```python
from build123d import *

# Parameters (mm, degrees)
SKETCH2_W                                   = 101.6
SKETCH2_H                                   = 127
BOSS_EXTRUDE1_DEPTH                         = 3.175
SKETCH5_R                                   = 3.9751
CUT_EXTRUDE1_DEPTH                          = 3.175
BOSS_EXTRUDE3_DEPTH                         = 92.87256
BOSS_EXTRUDE4_DEPTH                         = 6.35
SKETCH18_R                                  = 3.175
CUT_EXTRUDE3_DEPTH                          = 6.8072
FILLET4_R                                   = 4.0005
CUT_EXTRUDE4_DEPTH                          = 34.5948
CUT_EXTRUDE5_DEPTH                          = 2.9972
FILLET7_R                                   = 2.54
CSK_FOR_1_4_FLAT_HEAD_MACHINE_SCREW_2_COUNT = 2
CSK_FOR_1_4_FLAT_HEAD_MACHINE_SCREW_2_PITCH = 55.9


with BuildPart() as part:
    # Sketch2 → Boss-Extrude1 (new body)
    with BuildSketch(Plane.XY):
        with Locations((50.8, 63.5)):
            Rectangle(SKETCH2_W, SKETCH2_H)
    extrude(amount=BOSS_EXTRUDE1_DEPTH)

    # Sketch5 → Cut-Extrude1 (cut)
    with BuildSketch(Plane(origin=(0, 0, 0), x_dir=(-1, 0, 0), z_dir=(0, 0, -1))):
        with BuildLine():
            Line((-81.586228812, 65.152573183), (-58.571239337, 65.152573183))
            ThreePointArc((-58.571239337, 65.152573183), (-49.65943867, 58.729036089), (-53.287760408, 48.359981104))
            ThreePointArc((-53.287760408, 48.359981104), (-57.249364207, 28.049269577), (-36.93865268, 24.087665778))
            ThreePointArc((-36.93865268, 24.087665778), (-28.337713232, 24.971703827), (-22.817162059, 18.317291951))
            ThreePointArc((-22.817162059, 18.317291951), (-16.509170131, 7.896881921), (-5.03428, 3.81))
            Line((-5.03428, 3.81), (-5.03428, 0))
            Line((-5.03428, 0), (0, 0))
            Line((0, 0), (0, 127))
            Line((0, 127), (-101.6, 127))
            Line((-101.6, 127), (-101.6, 0))
            Line((-101.6, 0), (-97.90684, 0))
            Line((-97.90684, 0), (-97.90684, 65.152573183))
            Line((-97.90684, 65.152573183), (-81.586228812, 65.152573183))
        make_face()
        with Locations((-58.416247506, 55.973867932)):
            Circle(SKETCH5_R)
        with Locations((-31.810165582, 16.473778949)):
            Circle(SKETCH5_R)
    extrude(amount=-CUT_EXTRUDE1_DEPTH, mode=Mode.SUBTRACT)

    # Sketch10 → Boss-Extrude3 (add)
    with BuildSketch(Plane(origin=(5.03428, 0, 0), x_dir=(0, 0, -1), z_dir=(1, 0, 0))):
        Polygon((-3.175, 0), (-4.2418, 0), (-4.2418, -2.9972), (-34.5948, -2.9972), (-34.5948, 0), (-34.5948, 3.81), (-3.175, 3.81), align=None)
    extrude(amount=BOSS_EXTRUDE3_DEPTH)

    # Sketch11 → Boss-Extrude4 (add)
    with BuildSketch(Plane(origin=(97.90684, 0, 0), x_dir=(0, 0, -1), z_dir=(1, 0, 0))):
        Polygon((-3.175, 65.152573183), (-3.175, 3.81), (-34.5948, 3.81), align=None)
    extrude(amount=-BOSS_EXTRUDE4_DEPTH)

    # Sketch18 → Cut-Extrude3 (cut)
    with BuildSketch(Plane.XZ.offset(2.9972)):
        with Locations(Location((25.968032816, 23.228300068, 0), (0, 0, 270))):
            Circle(SKETCH18_R)
        with Locations(Location((81.868032816, 23.228300068, 0), (0, 0, 270))):
            Circle(SKETCH18_R)
    extrude(amount=-CUT_EXTRUDE3_DEPTH, mode=Mode.SUBTRACT)

    # Fillet4
    fillet4_edges = [part.edges().sort_by_distance(p)[0] for p in [
        (97.90684, -1.4986, 4.2418),
        (5.03428, -1.4986, 4.2418),
        (97.90684, 0.4064, 34.5948),
        (5.03428, 0.4064, 34.5948),
    ]]
    fillet(fillet4_edges, radius=FILLET4_R)

    # Mirror5: part across plane


with BuildPart() as part_1:
    add(part.part)
    add(part.part.mirror(Plane.XY))

    # Sketch25 → Cut-Extrude4 (cut)
    with BuildSketch(Plane.XY):
        Polygon((105.475480197, -15.241589329), (106.840773124, 71.833759528), (-8.541984089, 73.642896836), (-9.907277015, -13.432452021), align=None)
    extrude(amount=CUT_EXTRUDE4_DEPTH, mode=Mode.SUBTRACT)

    # Sketch28 → Cut-Extrude5 (cut)
    with BuildSketch(Plane.XZ.offset(2.9972)):
        with BuildLine():
            Line((93.90634, -4.2418), (9.03478, -4.2418))
            ThreePointArc((9.03478, -4.2418), (6.205999322, -5.413519322), (5.03428, -8.2423))
            Line((5.03428, -8.2423), (5.03428, -30.5943))
            ThreePointArc((5.03428, -30.5943), (6.205999322, -33.423080678), (9.03478, -34.5948))
            Line((9.03478, -34.5948), (93.90634, -34.5948))
            ThreePointArc((93.90634, -34.5948), (96.735120678, -33.423080678), (97.90684, -30.5943))
            Line((97.90684, -30.5943), (97.90684, -8.2423))
            ThreePointArc((97.90684, -8.2423), (96.735120678, -5.413519322), (93.90634, -4.2418))
        make_face()
    extrude(amount=-CUT_EXTRUDE5_DEPTH, mode=Mode.SUBTRACT)

    # Fillet7
    # the kernel refuses this fillet: 2.54 mm, written as the material it adds along each edge
    with BuildSketch(Plane(origin=(89.01684, 6.35, -5.715), x_dir=(0, -1, 0), z_dir=(1, 0, 0))) as fillet7_piece_1_section:
        Polygon((0, 0), (FILLET7_R, 0), (FILLET7_R, -FILLET7_R), (0, -FILLET7_R), align=None)
    fillet7_piece_1 = extrude(amount=FILLET7_R, mode=Mode.PRIVATE)
    fillet7_piece_1 = fillet7_piece_1 - Plane(origin=(89.01684, 6.35, -5.715), x_dir=(0, 0.7071067811865475, -0.7071067811865477), z_dir=(1, 0, 0)) * Sphere(FILLET7_R, mode=Mode.PRIVATE)
    add(fillet7_piece_1)
    with BuildSketch(Plane(origin=(5.03428, 3.81, -3.175), x_dir=(0, 0, -1), z_dir=(1, 0, 0))) as fillet7_piece_2_section:
        with BuildLine():
            CenterArc((FILLET7_R, FILLET7_R), FILLET7_R, 180, 90)
            Line((0, FILLET7_R), (0, 0))
            Line((0, 0), (FILLET7_R, 0))
        make_face()
    fillet7_piece_2 = extrude(amount=83.98256, mode=Mode.PRIVATE)
    fillet7_piece_2 = fillet7_piece_2 - Plane(origin=(5.03428, 21.962678524, -3.760034689), x_dir=(0.9796285454928902, -0.20081810888334822, 0), z_dir=(0, 0, -1)) * Cylinder(18.152678524, 179, mode=Mode.PRIVATE)
    add(fillet7_piece_2)
    with BuildSketch(Plane(origin=(91.55684, 3.81, -5.715), x_dir=(-1, 0, 0), z_dir=(0, 0, -1))) as fillet7_piece_3_section:
        with BuildLine():
            CenterArc((FILLET7_R, FILLET7_R), FILLET7_R, 180, 90)
            Line((0, FILLET7_R), (0, 0))
            Line((0, 0), (FILLET7_R, 0))
        make_face()
    fillet7_piece_3 = extrude(amount=28.8798, mode=Mode.PRIVATE)
    fillet7_piece_3 = split(fillet7_piece_3, bisect_by=Plane(origin=(90.978646613, 10.179733651, -31.332208508), z_dir=(0, -0.4558808495345019, 0.8900408142482573)), keep=Keep.TOP, mode=Mode.PRIVATE)
    add(fillet7_piece_3)
    with BuildSketch(Plane(origin=(91.55684, 65.152573183, -3.175), x_dir=(0, 0, -1), z_dir=(0, -1, 0))) as fillet7_piece_4_section:
        with BuildLine():
            CenterArc((FILLET7_R, -FILLET7_R), FILLET7_R, 90, 90)
            Line((0, -FILLET7_R), (0, 0))
            Line((0, 0), (FILLET7_R, 0))
        make_face()
    fillet7_piece_4 = extrude(amount=58.802573183, mode=Mode.PRIVATE)
    fillet7_piece_4 = split(fillet7_piece_4, bisect_by=Plane(origin=(90.975846211, 41.193986982, -15.446640195), z_dir=(0, -0.4558808495345019, 0.8900408142482573)), keep=Keep.TOP, mode=Mode.PRIVATE)
    add(fillet7_piece_4)

    # Sketch35 → CSK for 1/4 Flat Head Machine Screw (100)1 (revolve, cut)
    with BuildSketch(Plane(origin=(25.968032816, 3.81, -23.228300068), x_dir=(0, 0, 1), z_dir=(1, 0, 0))):
        Polygon((0, 0), (0, 3.81), (3.57124, 3.81), (3.57124, 3.298865467), (6.4389, 0), align=None)
    csk_for_1_4_flat_head_machine_screw_100 = revolve(axis=Axis((25.968032816, 10.16, -23.228300068), (0, -1, 0)), mode=Mode.SUBTRACT)

    # CSK for 1_4 Flat Head Machine Screw  2: CSK for 1/4 Flat Head Machine Screw (100)1 ×2
    with Locations(*[(i * CSK_FOR_1_4_FLAT_HEAD_MACHINE_SCREW_2_PITCH, 0, 0) for i in range(1, CSK_FOR_1_4_FLAT_HEAD_MACHINE_SCREW_2_COUNT)]):
        add(csk_for_1_4_flat_head_machine_screw_100, mode=Mode.SUBTRACT)


solid = part_1.part
```
Here's how the part is built. I have some questions about the finished solid (model axes, mm). A direction names the side the tool comes from. Coordinates: 2 decimals unless noted, no trailing zeros. Write each loop counter-clockwise with the first axis right and the second up, starting at its lowest first coordinate (ties: lowest second). Pieces come first, ordered by that corner, then holes. Notation, with made-up numbers: (-27, -39) -> (28, -39) arc R6 ccw to (28, -30) -> close; hole circle Ø1 at (82.5, 60). An arc over 180 degrees is marked (long way). Use a Markdown table: item, result. Add a question column.
(1) For faces 1 (the flat face through (91.557, 22, -13)), 2 (the flat face through (97.907, 26, -12)), which set-ups out of +Z, -Z, +X, -X, +Y, -Y let a thin tool reach every point of the face, with its end or its side?
(2) Please list where these lines run through material, in increasing order: line 1 (X direction, y = 3, z = -27); line 2 (Z direction, x = 52.5, y = 61.5) (3 decimals); line 3 (Y direction, x = 57, z = -9.5).
(3) We'd pull the mould along X, two halves only. Please class faces 3 (the cylindrical face through (6.237, 1.878, -33.454)), 4 (the flat face through (51, 2, -34.595)), 5 (the cylindrical face through (57.426, 28.318, -1.565)): +X half, -X half, draft (parallel to the pull), parting line (faces both ways), or undercut.
(4) If we section it at A-A, the plane x = 67: Write out the boundary of the cut face in (y, z) (3 decimals).
(5) If we section it at C-C, the plane z = -13: Write out the boundary of the cut face in (x, y), and give its area (3 significant figures).
(6) If we section it at B-B, the plane y = 53: Write out the boundary of the cut face in (x, z) (3 decimals), and give its area (3 significant figures).
(7) If we section it at D-D, the plane z = -24.5: State how many separate pieces and enclosed holes the cut face has, and give its area (3 significant figures).
(8) I'm going to push flat-ended pins straight in: P1, Ø4, axis at x = 79, y = 30.5, coming from the -Z side (3 decimals); P2, Ø3, axis at x = 88.5, z = -17, coming from the +Y side; P3, Ø5, axis at y = 56, z = -3.5, coming from the -X side. Where does each tip first touch, or does it pass through?
Outcome:
| question | item | result |
|---|---|---|
| 1 | face 1 | -Z, -X, +Y |
| 1 | face 2 | +Z, -Z, +X, +Y, -Y |
| 2 | line 1 | x = 5.03 to 21.65, 30.29 to 77.55, 86.19 to 97.91 |
| 2 | line 2 | z = -3.175 to 0 |
| 2 | line 3 | y = 0 to 3.81 |
| 3 | face 3 | -X half |
| 3 | face 4 | draft |
| 3 | face 5 | undercut |
| 4 | outline | (0, -34.595) -> (3.81, -34.595) -> (3.81, -5.715) arc R2.54 cw to (6.35, -3.175) -> (65.153, -3.175) -> (65.153, 0) -> (0, 0) -> close |
| 5 | outline | (5.03, 0) -> (97.91, 0) -> (97.91, 45.97) -> (91.56, 45.97) -> (91.56, 6.35) arc R2.54 cw to (89.02, 3.81) -> (5.03, 3.81) -> close |
| 5 | area | 623 mm^2 |
| 6 | outline | (49.731, -3.175) -> (55.779, -3.175) -> (55.779, 0) -> (49.731, 0) -> close; (61.054, -3.175) -> (89.017, -3.175) arc R2.54 cw to (91.557, -5.715) -> (91.557, -9.4) -> (97.907, -9.4) -> (97.907, 0) -> (61.054, 0) -> close |
| 6 | area | 177 mm^2 |
| 7 | separate pieces | 3 |
| 7 | enclosed holes | 0 |
| 7 | area | 410 mm^2 |
| 8 | P1 | stops at z = -3.175 |
| 8 | P2 | stops at y = 4.01 |
| 8 | P3 | stops at x = 49.24 |
